Geometry: final body of the model. Coordinates: model frame, mm. A direction names the side the tool comes from. Coordinates: 2 decimals unless noted, no trailing zeros. Order: outer loops, then holes, each group sorted by start corner. A loop starts at its lowest first (then second) coordinate and runs counter-clockwise, first axis right, second up. Notation, with made-up numbers: (76, 56.5) - (99, 56.5) arc R10 ccw to (99, 70.5) - close; hole circle Ø8 at (25, 75). An arc over 180 degrees is marked (long way). Use a Markdown table: item, result. Add a question column.
Autodesk Inventor part; units mm, degrees
ref_plane "Pracovní rovina1" through (0, 2.75, 0) normal (0, 1, 0) x (-1, 0, 0)
ref_plane "YZ Plane" through (0, 0, 0) normal (1, 0, 0) x (0, 1, 0)
ref_plane "XY Plane" through (0, 0, 0) normal (0, 0, 1) x (1, 0, 0)
sketch "Náčrt2" plane through (0, 0, 0) normal (1, 0, 0) x (0, 1, 0)
  line L0 (-2.5936, 18.2) -> (2.6216, 18.2)
  line L1 (-6.458, 6.9989) -> (0.6548, 6.9989)
  line L2 (-3.5412, 9.6623) -> (3.7182, 9.6623)
  line L3 (0, 18.2) -> (0, 9.6623)
  arc A0 (-2.5936, 18.2) -> (-3.5412, 9.6623) centre (0.0066, 13.59) ccw
  line L4 (0, 18.2) -> (0, 0)
revolve "Rotace1" add sketch "Náčrt2" angle 360 about axis through (0, 0, 18.2) along (0, 0, -1)
sketch "Náčrt3" plane through (0, 0, 18.2) normal (0, 0, 1) x (1, 0, 0)
  circle A0 centre (0, 0) radius 2
  dimension "d1" = 4
extrude "Vysunutí1" cut sketch "Náčrt3" against normal blind 10
sketch "Náčrt4" plane through (-3.5364, -0.0875, 0) normal (0, 0, -1) x (-1, 0, 0)
  circle A0 centre (-3.5364, 0.0875) radius 3.5412
  circle A1 centre (-3.5364, 0.0875) radius 2
  line L0 (-2.6864, -5.5125) -> (-2.6864, -3.3464)
  circle A2 centre (-3.5364, -5.5125) radius 0.85
  line L1 (-4.3864, -3.3464) -> (-4.3864, -5.5125)
  point P0 (-3.5364, 0.0875)
  point P1 (-4.3864, -3.3502)
  point P2 (-2.6864, -3.3502)
extrude "Vysunutí2" add sketch "Náčrt4" against normal blind 10 contours A0
sketch "Náčrt5" plane through (-3.5364, -0.0875, 0) normal (0, 0, -1) x (-1, 0, 0)
  point P0 (-3.5364, 0.0875)
extrude "Vysunutí3" add sketch "Náčrt4" against normal blind 7 contours A0 L0 A2 L1 | A2
sketch "Náčrt6" plane through (0, 0, 0) normal (0, 1, 0) x (-1, 0, 0)
  line L0 (0, 0) -> (-1.2, 0)
  line L1 (2, 0) -> (-2, 0)
  line L2 (-1.2, 0) -> (-1.2, 7.5)
  line L3 (-1.2, 7.5) -> (1.2, 7.5)
  line L4 (1.2, 7.5) -> (1.2, 0)
  arc A0 (1.2, 7.5) -> (-1.2, 7.5) centre (0, 7.5) ccw
  line L5 (0, 0) -> (1.2, 0)
  line L6 (-1.2, 7.5) -> (1.2, 7.5)
  line L7 (-1.2, 0) -> (1.2, 0)
  line L8 (1.2, 7.5) -> (1.2, 0)
  line L9 (1.2, 7.5) -> (-1.2, 7.5)
  line L10 (-1.2, 7.5) -> (-1.2, 0)
  dimension "d11" = 1.2
  dimension "d12" = 7.5
  dimension "d13" = 2.4
ref_plane "Pracovní rovina1" through (0, 2.75, 0) normal (0, 1, 0) x (-1, 0, 0)
sketch "Náčrt7" plane through (0, 0, 0) normal (0, 1, 0) x (-1, 0, 0)
  line L0 (1.2, 7.447) -> (1.2, 0)
  line L1 (-1.2, 7.447) -> (1.2041, 7.447)
  line L2 (1.2041, 7.447) -> (1.2041, 7.4445)
  line L3 (-1.2, 7.4445) -> (-1.2, 7.447)
  line L4 (1.2, 7.4445) -> (1.2, 0)
  line L5 (1.2, 0) -> (-1.2, 0)
  ellipse E0 centre (0.0021, 7.4458) end of major axis (0.0038, 9.0631) minor radius 1.2021 (1.2041, 7.4445) -> (-1.2, 7.4355) ccw
  line L6 (1.2, 7.4445) -> (1.2, 7.447)
  line L7 (1.2, 7.447) -> (-1.2, 7.447)
  line L8 (-1.2, 7.447) -> (-1.2, 7.4445)
  line L9 (-1.2, 0) -> (1.2041, 0)
  line L10 (1.2041, 0) -> (1.2041, 7.447)
  line L11 (1.2041, 7.447) -> (-1.2, 7.447)
  line L12 (-1.2, 7.447) -> (-1.2, 0)
  point P0 (0, 0)
  dimension "d9" = 2.4
  dimension "d10" = 7.447
extrude "Vysunutí4" cut sketch "Náčrt6" along normal blind 10
sketch "Náčrt8" plane through (-3.5364, -0.0875, 7) normal (0, 0, 1) x (1, 0, 0)
  arc A0 (2.6864, -5.5125) -> (4.3864, -5.5125) centre (3.5364, -5.5125) ccw
  line L0 (2.6864, -3.3502) -> (2.6864, -5.5125)
  line L1 (4.3864, -5.5125) -> (4.3864, -3.3502)
  arc A1 (4.3864, -3.3502) -> (2.6864, -3.3502) centre (3.5364, 0.0875) ccw
  arc A2 (4.3864, -3.3502) -> (4.7364, 3.4192) centre (3.5364, 0.0875) ccw
  arc A3 (2.3364, 1.6875) -> (4.7364, 1.6875) centre (3.5364, 0.0875) ccw
  circle A4 centre (3.5422, -2.8248) radius 3.5391
  line L2 (4.3864, -3.3502) -> (4.3864, -5.5125)
  arc A5 (2.6864, -5.5125) -> (4.3864, -5.5125) centre (3.5364, -5.5125) ccw
  line L3 (2.6864, -5.5125) -> (2.6864, -3.3502)
  line L4 (7.0813, -2.8203) -> (7.0776, 0.092)
  line L5 (0.003, -2.8342) -> (-0.0048, 0.078)
  line L6 (2.6864, -5.5125) -> (2.6864, -3.3502)
  arc A6 (2.6864, -5.5125) -> (4.3864, -5.5125) centre (3.5364, -5.5125) ccw
  arc A7 (2.3364, 3.4192) -> (2.6864, -3.3502) centre (3.5364, 0.0875) ccw
  line L7 (4.3864, -3.3502) -> (4.3864, -5.5125)
  arc A8 (2.6864, -5.5125) -> (4.3864, -5.5125) centre (3.5364, -5.5125) ccw
  line L8 (2.6864, -5.5125) -> (2.6864, -3.3502)
  arc A9 (2.3364, 1.6875) -> (4.7364, 1.6875) centre (3.5364, 0.0875) ccw
  line L9 (4.7364, 1.6875) -> (4.7364, 3.4192)
  arc A10 (4.3864, -3.3502) -> (4.7364, 3.4192) centre (3.5364, 0.0875) ccw
  line L10 (2.3364, 3.4192) -> (2.3364, 1.6875)
  line L11 (4.7364, 1.6875) -> (4.7364, 3.4192)
  arc A11 (2.3364, 3.4192) -> (2.6864, -3.3502) centre (3.5364, 0.0875) ccw
  line L12 (2.3364, 3.4192) -> (2.3364, 1.6875)
  point P0 (3.5364, 0.0875)
  point P1 (7.0776, 0.092)
  point P2 (-0.0048, 0.078)
extrude "Vysunutí5" add sketch "Náčrt8" against normal blind 1 contours A0 A4 A1 L0 | A0 L1 A1 A4 | L5 A1 A4 | A4 A1 L4
sketch "Náčrt9" plane through (-3.5364, -0.0875, 0) normal (0, 0, -1) x (-1, 0, 0)
  circle A0 centre (-3.5364, 0.0875) radius 2
  circle A1 centre (-3.5364, 0.0875) radius 3.5412
  circle A2 centre (-3.5364, -5.5125) radius 0.85
  line L0 (-4.3864, -5.5125) -> (-4.3864, -3.3502)
  line L1 (-2.6864, -5.5125) -> (-2.6864, -3.3502)
  line L2 (-4.7364, 1.6875) -> (-4.7364, 3.4192)
  line L3 (-2.3364, 1.6875) -> (-2.3364, 3.4192)
  point P0 (-3.5364, 0.0875)
properties part number "New_11_Base_Joint"
1) Section query A-A (z = 3.5). Return the cut outline in (x, y), and give its area (3 significant figures).
2) First-contact query: pin 1 (3 mm diameter, centred on x = -1, y = -5, fed in from +Z); pin 2 (1.1 mm diameter, centred on y = -4.5, z = 3.5, fed in from +X); pin 3 (0.5 mm diameter, centred on y = 2.5, z = 4, fed in from +X); pin 4 (3 mm diameter, centred on x = 0, y = 0, fed in from -Z). Flat tips, straight axial feed; report the tip coordinate or a pass-through.
3) Line query: line 1 (X direction, y = 0, z = 8.75); line 2 (Z direction, x = -2.75, y = -5); line 3 (Y direction, x = 0, z = 8.5). Output: solid intervals per line, ascending. Write a range as from..to.
4) Draft query along Y for faces 5 (the flat face through (1.2, 2, 4)), 6 (the cylindrical face through (0.02, -6.45, 2.96)), 7 (the cylindrical face through (0, 2, 9)). Return one class per face: released by +Y, released by -Y, zero draft, split by the parting line, or undercut.
5) Access query for faces 1 (the flat face through (-0.85, -5, 3)), 2 (the flat face through (0.85, -5, 3)), 3 (the cylindrical face through (0, 2.6, 8.7)), 4 (the flat face through (0, -3, 0)). Directions: +Z, -Z, +X, -X, +Y, -Y. A direction counts if a zero-diameter tool reaches every point of the face in a straight line with its end or side. Return the directions, or none.
From the geometry:
| question | item | result |
|---|---|---|
| 1 | outline | (-1.2, 1.6) - (-1.2, 3.33) arc R3.54 ccw to (-0.85, -3.44) - (-0.85, -5.6) arc R0.85 ccw to (0.85, -5.6) - (0.85, -3.44) arc R3.54 ccw to (1.2, 3.33) - (1.2, 1.6) arc R2 cw (long way) to start |
| 1 | area | 27.7 mm^2 |
| 2 | pin 1 | stops at z = 17.46 |
| 2 | pin 2 | stops at x = 0.85 |
| 2 | pin 3 | stops at x = 2.73 |
| 2 | pin 4 | passes through |
| 3 | line 1 | x = -3.54..-2, 2..3.54 |
| 3 | line 2 | z = 6..7 |
| 3 | line 3 | y = -3.54..-2 |
| 4 | face 5 | zero draft |
| 4 | face 6 | released by -Y |
| 4 | face 7 | undercut |
| 5 | face 1 | -Z, -X, -Y |
| 5 | face 2 | -Z, +X, -Y |
| 5 | face 3 | -Z, +Y |
| 5 | face 4 | -Z, +X, -X, +Y, -Y |
